Part model, mm, in its own coordinate system. Round coordinates to 2 decimals unless told otherwise and drop trailing zeros. Write each loop counter-clockwise with the first axis right and the second up, starting at its lowest first coordinate (ties: lowest second). Pieces come first, ordered by that corner, then holes. Notation, with made-up numbers: M 76,32.5 L 108,32.5 A6 cw 108,40.5 Z; hole C 22,-1 d9. An arc over 180 degrees is marked long. Use a Markdown table: item, result. Add a question column.
1) Wall check: probe 1 along Y at (x, z) = (-0.75, 1.3); probe 2 along Y at (x, z) = (0, 0.6); probe 3 along X at (y, z) = (-1.25, 0.4). Give the ranges that are in metal, low to high.
2) Slice it at A-A on z = 1.35. Write the cut outline in (x, y).
3) Two-plate mould, pull along Y, no slides. Class faces 1 (the face through (-1.5, 0.07, 0.89)), 2 (the face through (2.23, 1.38, 1.74)), 3 (the face through (2.31, -1.24, 1.74)): released by +Y, released by -Y, zero draft, split by the parting line, or undercut.
```python
from build123d import *

# Parameters (mm, degrees)
SKETCH_1_R      = 1.5
EXTRUDE_1_DEPTH = 1.8
FILLET_2_R      = 0.2


with BuildPart() as part:
    # 草图1 → 凸台-拉伸1 (new body)
    with BuildSketch(Plane.XY):
        Polygon((-1.487983369, -2.713381438), (1.605865571, -2.645322117), (3.09384894, 0.068059321), (1.487983369, 2.713381438), (-1.605865571, 2.645322117), (-3.09384894, -0.068059321), align=None)
        Circle(SKETCH_1_R, mode=Mode.SUBTRACT)
    extrude(amount=EXTRUDE_1_DEPTH)

    # 圆角2
    fillet_2_edges = [part.edges().sort_by_distance(p)[0] for p in [
        (2.349857255, -1.288631398, 1.8),
        (-3.09384894, -0.068059321, 0.9),
        (-1.605865571, 2.645322117, 0.9),
        (1.487983369, 2.713381438, 0.9),
        (3.09384894, 0.068059321, 0.9),
        (1.605865571, -2.645322117, 0.9),
        (-1.487983369, -2.713381438, 0.9),
        (2.290916154, 1.390720379, 1.8),
        (-0.058941101, 2.679351777, 1.8),
        (-2.349857255, 1.288631398, 1.8),
        (-2.290916154, -1.390720379, 1.8),
        (-2.349857255, 1.288631398, 0),
        (-0.058941101, 2.679351777, 0),
        (2.290916154, 1.390720379, 0),
        (0.058941101, -2.679351777, 1.8),
        (2.349857255, -1.288631398, 0),
        (0.058941101, -2.679351777, 0),
        (-2.290916154, -1.390720379, 0),
    ]]
    fillet(fillet_2_edges, radius=FILLET_2_R)


solid = part.part
```
Entries:
| question | item | result |
|---|---|---|
| 1 | probe 1 | y = -2.7 to -1.3, 1.3 to 2.66 |
| 1 | probe 2 | y = -2.68 to -1.5, 1.5 to 2.68 |
| 1 | probe 3 | x = -2.38 to -0.83, 0.83 to 2.37 |
| 2 | outline | M -3.04,0.03 A0.2 ccw -3.03,-0.17 L -1.55,-2.61 A0.2 ccw -1.37,-2.71 L 1.49,-2.65 A0.2 ccw 1.66,-2.54 L 3.04,-0.03 A0.2 ccw 3.03,0.17 L 1.55,2.61 A0.2 ccw 1.37,2.71 L -1.49,2.65 A0.2 ccw -1.66,2.54 Z; hole C 0,0 d3 |
| 3 | face 1 | undercut |
| 3 | face 2 | released by +Y |
| 3 | face 3 | released by -Y |
